Build history of the part. All positions in model axes, mm. A direction names the side the tool comes from. Round coordinates to 2 decimals unless told otherwise and drop trailing zeros. Write each loop counter-clockwise with the first axis right and the second up, starting at its lowest first coordinate (ties: lowest second). Pieces come first, ordered by that corner, then holes. Notation, with made-up numbers: (28.5, -1) -> (48.5, -1) arc R19 ccw to (48.5, 29) -> close; hole circle Ø6 at (27, 70.5). An arc over 180 degrees is marked (long way). Answer in a Markdown table with one row per item.
Autodesk Inventor part; units mm, degrees
ref_plane "작업 평면1" through (0, -6, 0) normal (0, -1, 0) x (1, 0, 0)
ref_plane "YZ Plane" through (0, 0, 0) normal (1, 0, 0) x (0, 1, 0)
ref_plane "XZ Plane" through (0, 0, 0) normal (0, 1, 0) x (-1, 0, 0)
sketch "스케치1" plane through (0, 0, 0) normal (0, 1, 0) x (-1, 0, 0)
  circle A0 centre (0, 0) radius 18
  dimension "d0" = 36
extrude "돌출1" add sketch "스케치1" along normal blind 12.8
sketch "스케치5" plane through (0, 0, 0) normal (0, -1, 0) x (1, 0, 0)
  arc A0 (3.4721, 22.3558) -> (-3.4721, 22.3558) centre (0, 21.915) ccw
  arc A1 (-3.4721, -22.3558) -> (3.4721, -22.3558) centre (0, -21.915) ccw
  line L0 (0, 21.915) -> (0, -21.915) construction
  circle A2 centre (0, 21.915) radius 1.25
  circle A3 centre (0, -21.915) radius 1.25
  arc A4 (3.4721, 22.3558) -> (7.8981, 16.1747) centre (11.4084, 23.3634) ccw
  arc A5 (7.8981, -16.1747) -> (3.4721, -22.3558) centre (11.4084, -23.3634) ccw
  arc A6 (-3.4721, -22.3558) -> (-7.8981, -16.1747) centre (-11.4084, -23.3634) ccw
  arc A7 (-7.8981, 16.1747) -> (-3.4721, 22.3558) centre (-11.4084, 23.3634) ccw
  circle A8 centre (0, 0) radius 18
  circle A9 centre (0, 0) radius 18
  dimension "d14" = 7
  dimension "d15" = 7
  dimension "d16" = 43.83
  dimension "d17" = 2.5
  dimension "d18" = 2.5
  dimension "d19" = 16
  dimension "d20" = 16
  dimension "d21" = 16
  dimension "d22" = 16
extrude "돌출4" add sketch "스케치5" along normal blind 2.5
thread "스레드1"
thread "스레드2"
sketch "스케치6" plane through (0, -2.5, 0) normal (0, -1, 0) x (1, 0, 0)
  circle A0 centre (0, 0) radius 8
  dimension "d29" = 16
extrude "돌출5" add sketch "스케치6" along normal blind 1.85
ref_plane "작업 평면1" through (0, -6, 0) normal (0, -1, 0) x (1, 0, 0)
sketch "스케치7" plane through (0, -4.35, 0) normal (0, -1, 0) x (1, 0, 0)
  circle A0 centre (0, 0) radius 2.5
  dimension "d33" = 5
extrude "돌출6" add sketch "스케치7" along normal blind 7.65
sketch "스케치9" plane through (0, 0, 0) normal (0, 0, 1) x (1, 0, 0)
  line L0 (-2.5, -12) -> (2.5, -12)
  line L1 (2.5, -12) -> (6.8309, -12)
  line L2 (6.8309, -12) -> (6.8309, -7.4987)
  line L3 (6.8309, -7.4987) -> (7.3309, -7.4987)
  line L4 (2.5, -4.35) -> (2.5, -12)
  line L5 (7.3309, -7.4987) -> (7.3309, -5.9987)
  line L6 (7.3309, -5.9987) -> (2.5, -5.9987)
  line L7 (0, -13.2553) -> (0, -2.7284)
  point P0 (0, 0)
  dimension "d36" = 1.5
  dimension "d37" = 0.5
revolve "회전1" add sketch "스케치9" angle 360 about axis through (0, -13.2553, 0) along (0, 1, 0)
properties part number "스텝모터"
Q1. Saw through at C-C on z = 17. Write the cut outline in (x, y), plus the area to 3 significant figures.
A:
| item | result |
|---|---|
| outline | (-6.56, -2.5) -> (6.56, -2.5) -> (6.56, 0) -> (5.92, 0) -> (5.92, 12.8) -> (-5.92, 12.8) -> (-5.92, 0) -> (-6.56, 0) -> close |
| area | 184 mm² |
Q2. Saw through at A-A on x = 0. State how many separate pieces and enclosed holes the cut face has, plus the area to 3 significant figures.
A:
| item | result |
|---|---|
| separate pieces | 3 |
| enclosed holes | 0 |
| area | 697 mm² |
Q3. Two-plate mould, pull along Z, no slides. Class faces 4 (the cylindrical face through (-0.3, -1.2, -20.7)), 5 (the cylindrical face through (0.67, -1.23, 20.86)), 6 (the flat face through (0, 0, 20)), 7 (the cylindrical face through (-0.95, -6.74, -7.27)): released by +Z, released by -Z, zero draft, split by the parting line, or undercut.
A:
| item | result |
|---|---|
| face 4 | undercut |
| face 5 | undercut |
| face 6 | zero draft |
| face 7 | split by the parting line |
Q4. Saw through at D-D on y = -5. Write the cut outline in (x, z).
A:
| item | result |
|---|---|
| outline | circle Ø5 at (0, 0) |
Q5. Saw through at B-B on x = -6. Write the cut outline in (y, z).
A:
| item | result |
|---|---|
| outline | (-12, -3.27) -> (-7.5, -3.27) -> (-7.5, -4.21) -> (-6, -4.21) -> (-6, 4.21) -> (-7.5, 4.21) -> (-7.5, 3.27) -> (-12, 3.27) -> close; (-4.35, -5.29) -> (-2.5, -5.29) -> (-2.5, -17.47) -> (0, -17.47) -> (0, -16.97) -> (12.8, -16.97) -> (12.8, 16.97) -> (0, 16.97) -> (0, 17.47) -> (-2.5, 17.47) -> (-2.5, 5.29) -> (-4.35, 5.29) -> close |
Q6. Wall check: line 1 (Z direction, x = 0, y = -1.8) (3 decimals); line 2 (Y direction, x = 3, z = 3.5); line 3 (Y direction, x = 16, z = 4). Give the ranges that are in metal, low to high. Write a range as [from, to].
A:
| item | result |
|---|---|
| line 1 | [-25.415, -23.165], [-20.665, 20.665], [23.165, 25.415] |
| line 2 | [-12, -6], [-4.35, 12.8] |
| line 3 | [-2.5, 12.8] |
Q7. Drop flat-ended pins along their axis: P1, Ø4, axis at x = 0, z = -21.915, coming from the +Y side; P2, Ø8, axis at x = 6.5, y = -1.5, coming from the +Z side; P3, Ø1.5, axis at y = -6, z = 0, coming from the -X side. Give the stop position or say it passes through.
A:
| item | result |
|---|---|
| P1 | y = 0 |
| P2 | z = 24.36 |
| P3 | x = -7.33 |
Q8. Which spindle directions (+Z, -Z, +X, -X, +Y, -Y) get a long thin tool onto all of the face, cutting with end or side? Do faces 1 (the flat face through (3, -5.999, 0)), 2 (the flat face through (5, -7.499, 5)), 3 (the cylindrical face through (-4.936, -1.232, -18.661)). Say none if no direction does.
A:
| item | result |
|---|---|
| face 1 | none |
| face 2 | -Y |
| face 3 | -Z, -X, +Y, -Y |
